```python
from build123d import *

# Parameters (mm, degrees)
SKETCH_1_R          = 2.95
EXTRUDE_1_DEPTH     = 2.7
SKETCH_2_R          = 1.25
EXTRUDE_2_DEPTH     = 30
SKETCH_3_R          = 1
EXTRUDE_3_DEPTH     = 4
CUT_EXTRUDE_1_DEPTH = 2
FILLET_1_R          = 0.2


with BuildPart() as part:
    # 草图1 → 凸台-拉伸1 (new body)
    with BuildSketch(Plane(origin=(0, 0, 0), x_dir=(1, 0, 0), z_dir=(0, 1, 0))):
        Circle(SKETCH_1_R)
    extrude(amount=EXTRUDE_1_DEPTH)

    # 草图2 → 凸台-拉伸2 (add)
    with BuildSketch(Plane(origin=(0, 2.7, 0), x_dir=(1, 0, 0), z_dir=(0, 1, 0))):
        Circle(SKETCH_2_R)
    extrude(amount=EXTRUDE_2_DEPTH)

    # 草图3 → 凸台-拉伸3 (add)
    with BuildSketch(Plane(origin=(0, 32.7, 0), x_dir=(1, 0, 0), z_dir=(0, 1, 0))):
        Circle(SKETCH_3_R)
    extrude(amount=EXTRUDE_3_DEPTH)

    # 草图4 → 切除-拉伸1 (cut)
    with BuildSketch(Plane.XZ):
        Polygon((2.247285488, -0.53201623), (1.584382314, 1.680198207), (-0.662903174, 2.212214437), (-2.247285488, 0.53201623), (-1.584382314, -1.680198207), (0.662903174, -2.212214437), align=None)
    extrude(amount=-CUT_EXTRUDE_1_DEPTH, mode=Mode.SUBTRACT)

    # 圆角1
    fillet_1_edges = [part.edges().sort_by_distance(p)[0] for p in [
        (-1, 36.7, 0),
        (-2.95, 0, 0),
        (-2.95, 2.7, 0),
    ]]
    fillet(fillet_1_edges, radius=FILLET_1_R)


solid = part.part
```
Read the model definition and answer for the solid it produces. Units are mm, in the model's axes. A direction names the side the tool comes from. Coordinates: 2 decimals unless noted, no trailing zeros. Write each loop counter-clockwise with the first axis right and the second up, starting at its lowest first coordinate (ties: lowest second). Pieces come first, ordered by that corner, then holes. Notation, with made-up numbers: (54, 15) -> (91, 15) arc R20 ccw to (91, 33) -> close; hole circle Ø4 at (21.5, -33.5). An arc over 180 degrees is marked (long way). Answer as a JSON object with one key per item and string values.
Q1. Flat-ended cylindrical pins translate along their axes: pin 1 Ø1.5 at (x, y) = (-1, 8) entering from -Z; pin 2 Ø1.5 at (y, z) = (19.5, 1) entering from +X; pin 3 Ø1.3 at (x, z) = (1, 0.5) entering from -Y; pin 4 Ø2 at (x, z) = (1, -1.5) entering from -Y. Find the tip coordinate at first contact, or state that the pin passes through.
The answers:
{"pin 1": "stops at z = -1.22", "pin 2": "stops at x = 1.22", "pin 3": "stops at y = 2", "pin 4": "stops at y = 0"}
Q2. A tool of negligible diameter and unlimited length cuts with its end or side. For faces 1 (the flat face through (1, 2.7, 1)), 2 (the flat face through (1.92, 0.99, 0.56)), 3 (the flat face through (-2, 0, -1)), from which of +Z, -Z, +X, -X, +Y, -Y can it reach the whole face along a straight path? Write none if from no direction.
The answers:
{"face 1": "+Y", "face 2": "-Y", "face 3": "+Z, -Z, +X, -X, -Y"}
Q3. The part is cut by section A-A on y = 10.5. Give the vertices of the cut face in (x, z).
The answers:
{"outline": "circle Ø2.5 at (0, 0)"}
Q4. The part is cut by section B-B on x = 0. Give the vertices of the cut face in (y, z).
The answers:
{"outline": "(0, -2.75) arc R0.2 ccw to (0.2, -2.95) -> (2.5, -2.95) arc R0.2 ccw to (2.7, -2.75) -> (2.7, -1.25) -> (32.7, -1.25) -> (32.7, -1) -> (36.5, -1) arc R0.2 ccw to (36.7, -0.8) -> (36.7, 0.8) arc R0.2 ccw to (36.5, 1) -> (32.7, 1) -> (32.7, 1.25) -> (2.7, 1.25) -> (2.7, 2.75) arc R0.2 ccw to (2.5, 2.95) -> (0.2, 2.95) arc R0.2 ccw to (0, 2.75) -> (0, 2.06) -> (2, 2.06) -> (2, -2.06) -> (0, -2.06) -> close"}
Q5. Determine the mould class of faces 4 (the cylindrical face through (-0.27, 17.49, 1.22)), 5 (the flat face through (0, 36.7, 0)), 6 (the flat face through (0.48, 0.99, 1.94)) for opening direction Z: pulls with the +Z half, pulls with the -Z half, needs draft (parallel to the pull), parting line crosses it, or undercut.
The answers:
{"face 4": "parting line crosses it", "face 5": "needs draft", "face 6": "undercut"}
Q6. Consider line 1 (Y direction, x = -0.2, z = 0.75); line 2 (Y direction, x = -0.25, z = 2.55); line 3 (X direction, y = 20.5, z = -1). Determine where each line is inside the solid, lowest interval first. Write a range as [from, to].
The answers:
{"line 1": "y = [2, 36.7]", "line 2": "y = [0, 2.7]", "line 3": "x = [-0.75, 0.75]"}
Q7. The part is cut by section C-C on z = 0. Give the vertices of the cut face in (x, y), then the cut area to 3 significant figures.
The answers:
{"outline": "(-2.95, 0.2) arc R0.2 ccw to (-2.75, 0) -> (-2.09, 0) -> (-2.09, 2) -> (2.09, 2) -> (2.09, 0) -> (2.75, 0) arc R0.2 ccw to (2.95, 0.2) -> (2.95, 2.5) arc R0.2 ccw to (2.75, 2.7) -> (1.25, 2.7) -> (1.25, 32.7) -> (1, 32.7) -> (1, 36.5) arc R0.2 ccw to (0.8, 36.7) -> (-0.8, 36.7) arc R0.2 ccw to (-1, 36.5) -> (-1, 32.7) -> (-1.25, 32.7) -> (-1.25, 2.7) -> (-2.75, 2.7) arc R0.2 ccw to (-2.95, 2.5) -> close", "area": "90.5 mm2"}
